```python
from build123d import *

# Parameters (mm, degrees)
BOSS_EXTRUDE1_DEPTH = 101.6
SKETCH2_W           = 4.7625
SKETCH2_H           = 38.1
SKETCH2_H_2         = 35.194001629
BOSS_EXTRUDE2_DEPTH = 44.45
FILLET1_R           = 19.05
FILLET4_R           = 2.54
FILLET5_R           = 2.54
SKETCH4_R           = 1.190625
CUT_EXTRUDE1_DEPTH  = 128.07291971
SKETCH5_R           = 1.5875
SKETCH5_W           = 19.84375
SKETCH5_H           = 39.6875
CUT_EXTRUDE2_DEPTH  = 117.05035969
SKETCH6_R           = 6.418083015
SKETCH6_R_2         = 2.38125
BOSS_EXTRUDE3_DEPTH = 7.9375
SKETCH7_R           = 2.38125
CUT_EXTRUDE3_DEPTH  = 117.05035969
CUT_EXTRUDE4_START  = -12.7
SKETCH8_R           = 1.190625
SKETCH8_R_2         = 2.38125
CUT_EXTRUDE4_DEPTH  = 12.7
CUT_EXTRUDE5_DEPTH  = 2.38125
SKETCH10_R          = 6.731
CUT_EXTRUDE6_DEPTH  = 127.239951738
CUT_EXTRUDE7_DEPTH  = 129.848153517


with BuildPart() as part:
    # Sketch1 → Boss-Extrude1 (new body)
    with BuildSketch(Plane.XY):
        Polygon((-36.065906398, 24.64981637), (36.165343602, 24.64981637), (36.165343602, -15.306685259), (31.402843602, -15.306685259), (31.402843602, 19.88731637), (-31.303406398, 19.88731637), (-31.303406398, -18.21268363), (-36.065906398, -18.21268363), align=None)
    extrude(amount=BOSS_EXTRUDE1_DEPTH)

    # Sketch2 → Boss-Extrude2 (add)
    with BuildSketch(Plane(origin=(0, 0, 0), x_dir=(-1, 0, 0), z_dir=(0, 0, -1))):
        with Locations((33.684656398, 0.83731637)):
            Rectangle(SKETCH2_W, SKETCH2_H)
        with Locations((-33.784093602, 2.290315555)):
            Rectangle(SKETCH2_W, SKETCH2_H_2)
    extrude(amount=BOSS_EXTRUDE2_DEPTH)

    # Fillet1
    # the kernel refuses this fillet: 19.05 mm, written as the material it takes off along each edge
    with BuildSketch(Plane(origin=(16.321593602, -18.21268363, -44.45), x_dir=(0, 0, 1), z_dir=(-1, 0, 0))) as fillet1_piece_1:
        with BuildLine():
            CenterArc((FILLET1_R, FILLET1_R), FILLET1_R, 180, 90)
            Line((0, FILLET1_R), (0, 0))
            Line((0, 0), (FILLET1_R, 0))
        make_face()
    extrude(amount=100.0125, mode=Mode.SUBTRACT)
    with BuildSketch(Plane(origin=(-83.690906398, 19.88731637, -44.45), x_dir=(0, -1, 0), z_dir=(1, 0, 0)), Plane(origin=(83.790343602, -15.306685259, -44.45), x_dir=(0, 1, 0), z_dir=(-1, 0, 0)), Plane(origin=(-16.222156398, 19.88731637, -44.45), x_dir=(0, -1, 0), z_dir=(1, 0, 0))) as fillet1_piece_2:
        with BuildLine():
            CenterArc((FILLET1_R, -FILLET1_R), FILLET1_R, 90, 90)
            Line((0, -FILLET1_R), (0, 0))
            Line((0, 0), (FILLET1_R, 0))
        make_face()
    extrude(amount=100.0125, mode=Mode.SUBTRACT)

    # Fillet4
    fillet4_edges = [part.edges().sort_by_distance(p)[0] for p in [
        (-36.065906398, 24.64981637, 50.8),
        (36.165343602, 24.64981637, 50.8),
        (31.402843602, 19.88731637, 50.8),
        (-31.303406398, 19.88731637, 50.8),
    ]]
    fillet(fillet4_edges, radius=FILLET4_R)

    # Fillet5
    fillet5_edges = [part.edges().sort_by_distance(p)[0] for p in [
        (33.784093602, -15.306685259, 101.6),
        (-33.684656398, -18.21268363, 101.6),
    ]]
    fillet(fillet5_edges, radius=FILLET5_R)

    # Sketch4 → Cut-Extrude1 (cut, through all)
    with BuildSketch(Plane.ZY.offset(36.065906398)):
        with Locations((-25.4, 0.83731637)):
            Circle(SKETCH4_R)
        with Locations((0, 0.83731637)):
            Circle(SKETCH4_R)
    extrude(amount=-CUT_EXTRUDE1_DEPTH, mode=Mode.SUBTRACT)

    # Sketch5 → Cut-Extrude2 (cut, through all)
    with BuildSketch(Plane(origin=(0, 24.64981637, 0), x_dir=(1, 0, 0), z_dir=(0, 1, 0))):
        with Locations(Location((-22.298893396, -26.9875, 0), (0, 0, 270))):
            Circle(SKETCH5_R)
        with Locations(Location((-11.980143396, -26.9875, 0), (0, 0, 180))):
            Circle(SKETCH5_R)
        with Locations(Location((-11.980143396, -74.6125, 0), (0, 0, 270))):
            Circle(SKETCH5_R)
        with Locations(Location((-22.298893396, -74.6125, 0), (0, 0, 180))):
            Circle(SKETCH5_R)
        with Locations((-17.139518396, -50.8)):
            Rectangle(SKETCH5_W, SKETCH5_H)
    extrude(amount=-CUT_EXTRUDE2_DEPTH, mode=Mode.SUBTRACT)

    # Sketch6 → Boss-Extrude3 (add)
    with BuildSketch(Plane(origin=(0, 24.64981637, 0), x_dir=(1, 0, 0), z_dir=(0, 1, 0))):
        with Locations(Location((1.910481604, -61.11875, 0), (0, 0, 90))):
            Circle(SKETCH6_R)
        with Locations(Location((1.910481604, -61.11875, 0), (0, 0, 270))):
            Circle(SKETCH6_R_2, mode=Mode.SUBTRACT)
    extrude(amount=BOSS_EXTRUDE3_DEPTH)

    # Sketch7 → Cut-Extrude3 (cut, through all)
    with BuildSketch(Plane(origin=(0, 24.64981637, 0), x_dir=(1, 0, 0), z_dir=(0, 1, 0))):
        with Locations(Location((1.910481604, -61.11875, 0), (0, 0, 180))):
            Circle(SKETCH7_R)
    extrude(amount=-CUT_EXTRUDE3_DEPTH, mode=Mode.SUBTRACT)

    # Sketch8 → Cut-Extrude4 (cut)
    with BuildSketch(Plane(origin=(36.165343602, 0, 0), x_dir=(0, 0, -1), z_dir=(1, 0, 0)).offset(CUT_EXTRUDE4_START)):
        with Locations(Location((0, 0.83731637, 0), (0, 0, 180))):
            Circle(SKETCH8_R)
        with Locations(Location((25.4, 0.83731637, 0), (0, 0, 90))):
            Circle(SKETCH8_R_2)
    extrude(amount=CUT_EXTRUDE4_DEPTH, mode=Mode.SUBTRACT)

    # Sketch9 → Cut-Extrude5 (cut)
    with BuildSketch(Plane.ZY.offset(36.065906398)):
        with BuildLine():
            Line((-25.069295566, 6.097430896), (0.016544331, 4.520279211))
            ThreePointArc((0.016544331, 4.520279211), (3.683, 0.83731637), (0.016544331, -2.84564647))
            Line((0.016544331, -2.84564647), (-25.069295566, -4.422798156))
            ThreePointArc((-25.069295566, -4.422798156), (-30.6705, 0.83731637), (-25.069295566, 6.097430896))
        make_face()
    extrude(amount=-CUT_EXTRUDE5_DEPTH, mode=Mode.SUBTRACT)

    # Sketch10 → Cut-Extrude6 (cut, through all)
    with BuildSketch(Plane(origin=(-31.303406398, 0, 0), x_dir=(0, 0, -1), z_dir=(1, 0, 0))):
        with Locations((25.4, 0.83731637)):
            Circle(SKETCH10_R)
    extrude(amount=-CUT_EXTRUDE6_DEPTH, mode=Mode.SUBTRACT)

    # Sketch11 → Cut-Extrude7 (cut, through all)
    with BuildSketch(Plane.ZY.offset(36.065906398)):
        with BuildLine():
            Line((78.230942549, 28.285686863), (107.145035189, 28.285686863))
            Line((107.145035189, 28.285686863), (107.145035189, -25.578978537))
            Line((107.145035189, -25.578978537), (47.434592149, -25.578978537))
            Line((47.434592149, -25.578978537), (47.434592149, -18.811963789))
            ThreePointArc((47.434592149, -18.811963789), (77.401439504, -4.789344682), (78.230942549, 28.285686863))
        make_face()
    extrude(amount=-CUT_EXTRUDE7_DEPTH, mode=Mode.SUBTRACT)


solid = part.part
```
Geometry check sheet. Reference: the model listing, model coordinates, mm. A direction names the side the tool comes from. Give positions to 0.01 mm unless a question says otherwise; leave off trailing zeros. Write each loop counter-clockwise with the first axis right and the second up, starting at its lowest first coordinate (ties: lowest second). Pieces come first, ordered by that corner, then holes.
1) Access from +Z, -Z, +X, -X, +Y, -Y to the whole of each face (thin tool, end or side, straight path). Record for faces 1 (the cylindrical face through (33.75, 1.94, -27.51)), 2 (the flat face through (-7.218, 22, 51)), 3 (the cylindrical face through (-33.65, -1.74, -31.62)), 4 (the cylindrical face through (-30.6, 19.1, 41.6)), 5 (the cylindrical face through (-2.427, 28.563, 65.849)).
2) Section check C-C, the plane y = 13. Record the boundary of the cut face in (x, z), and give its area (3 significant figures).
3) Section check D-D, the plane z = 16.5. Record the boundary of the cut face in (x, y).
4) Material ranges on L1, parallel to X at y = -12.5, z = -22; L2, parallel to X at y = 21.5, z = 60.5; L3, parallel to Y at x = 23.5, z = 74.5, recorded low to high.
5) Release check for a two-part mould opening along Y. For faces 6 (the flat face through (-34.892, -3.494, -10.291)), 7 (the flat face through (-34, -18.213, 17)), 8 (the cylindrical face through (-13.389, 22.302, 75.345)) record: pulls with the +Y half, pulls with the -Y half, needs draft (parallel to the pull), parting line crosses it, or undercut.
6) Section check A-A, the plane x = -17.5. Record the boundary of the cut face in (y, z).
7) Gauge pin test, flat ends, axial feed: pin 1 (8 mm diameter, centred on x = 8.5, y = 22, fed in from +Z); pin 2 (1.4 mm diameter, centred on x = -20.5, y = 23, fed in from +Z); pin 3 (10 mm diameter, centred on x = 23, y = -2.5, fed in from -Z); pin 4 (12 mm diameter, centred on x = -26.5, z = -10.5, fed in from +Y). Record the tip position at first contact, or that the pin passes through.
8) Section check B-B, the plane z = 51.5. Record the boundary of the cut face in (x, y).
Computed:
1. face 1: +X, -X
1. face 2: +Y, -Y
1. face 3: -X
1. face 4: +Z, -Z, -Y
1. face 5: +Y
2. outline: (-36.07, -40.06) - (-31.3, -40.06) - (-31.3, 82.52) - (-36.07, 82.52) - close; (31.4, -40.06) - (36.17, -40.06) - (36.17, 82.52) - (31.4, 82.52) - close
2. area: 1,170 mm2
3. outline: (-36.07, -18.21) - (-31.3, -18.21) - (-31.3, 17.35) arc R2.54 cw to (-28.76, 19.89) - (28.86, 19.89) arc R2.54 cw to (31.4, 17.35) - (31.4, -15.31) - (36.17, -15.31) - (36.17, 22.11) arc R2.54 ccw to (33.63, 24.65) - (-33.53, 24.65) arc R2.54 ccw to (-36.07, 22.11) - close
4. L1: x = -36.07 to -31.3, 31.4 to 36.17
4. L2: x = -36.07 to -27.06, -7.22 to -0.39, 4.21 to 36.17
4. L3: y = 19.89 to 24.65
5. face 6: undercut
5. face 7: pulls with the -Y half
5. face 8: needs draft
6. outline: (19.89, 0) - (24.65, 0) - (24.65, 30.96) - (19.89, 30.96) - close; (19.89, 70.64) - (24.65, 70.64) - (24.65, 80.05) arc R31.44 ccw to (19.89, 81.63) - close
7. pin 1: stops at z = 81.63
7. pin 2: stops at z = 80.94
7. pin 3: passes through
7. pin 4: stops at y = 19.89
8. outline: (-36.07, -18.21) - (-31.3, -18.21) - (-31.3, 17.35) arc R2.54 cw to (-28.76, 19.89) - (-27.06, 19.89) - (-27.06, 24.65) - (-33.53, 24.65) arc R2.54 ccw to (-36.07, 22.11) - close; (-7.22, 19.89) - (28.86, 19.89) arc R2.54 cw to (31.4, 17.35) - (31.4, -15.31) - (36.17, -15.31) - (36.17, 22.11) arc R2.54 ccw to (33.63, 24.65) - (-7.22, 24.65) - close
